The listing builds one solid part. Answer for the finished solid, in the listing's coordinates (mm). A direction names the side the tool comes from. Give positions to 0.01 mm unless a question says otherwise; leave off trailing zeros. Loops run counter-clockwise (first coordinate to the right, second up) from the corner with the lowest first, then second, coordinate; pieces in that order, holes last.
Item 1: The mould has two halves that part along X. Classify faces 3 (the face through (22, 79, -70.679)), 4 (the face through (12, 76.072, -67)): pulls with the +X half, pulls with the -X half, needs draft (parallel to the pull), parting line crosses it, or undercut.
Item 2: Section A-A, the plane x = -18 is taken. Give the vertices of the cut face in (y, z), and give its area (3 significant figures).
Item 3: Each of these flat-tipped pins is pushed along its axis until it touches: pin 1 Ø3 at (x, y) = (32.47, 78.92) entering from +Z; pin 2 Ø1.7 at (x, y) = (62.5, 80) entering from +Z; pin 3 Ø4 at (x, y) = (13.5, 78) entering from +Z. Where does it stop, or does it pass through?
Item 4: A tool of negligible diameter and unlimited length cuts with its end or side. For faces 1 (the face through (12.12, 77.31, -69.3)), 2 (the face through (32, 76.072, -67)), from which of +Z, -Z, +X, -X, +Y, -Y can it reach the whole face along a straight path? Write none if from no direction.
Item 5: Consider line 1 along X through (y, z) = (79.5, -65.9); line 2 along X through (y, z) = (79, -67.25); line 3 along Y through (x, z) = (11, -68.55). Determine where each line is inside the solid, lowest interval first.
from build123d import *

# Parameters (mm, degrees)
SKETCH1_W           = 99.9
SKETCH1_H           = 24.9
SKETCH1_R           = 1.65
BOSS_EXTRUDE1_DEPTH = 5
CUT_EXTRUDE1_DEPTH  = 2.2


with BuildPart() as part:
    # Sketch1 → Boss-Extrude1 (new body)
    with BuildSketch(Plane.XY.offset(-70.679368873)):
        with Locations((22.473815584, 78.921604181)):
            Rectangle(SKETCH1_W, SKETCH1_H)
        with Locations((-17.526184416, 78.921604181)):
            Circle(SKETCH1_R, mode=Mode.SUBTRACT)
        with Locations((12.473815584, 78.921604181)):
            Circle(SKETCH1_R, mode=Mode.SUBTRACT)
        with Locations((32.473815584, 78.921604181)):
            Circle(SKETCH1_R, mode=Mode.SUBTRACT)
        with Locations((62.473815584, 78.921604181)):
            Circle(SKETCH1_R, mode=Mode.SUBTRACT)
    extrude(amount=BOSS_EXTRUDE1_DEPTH)

    # Sketch2 → Cut-Extrude1 (cut)
    with BuildSketch(Plane.XY.offset(-65.679368873)):
        Polygon((-15.880736149, 76.071604181), (-14.235287881, 78.921604181), (-15.880736149, 81.771604181), (-19.171632683, 81.771604181), (-20.81708095, 78.921604181), (-19.171632683, 76.071604181), align=None)
        Polygon((14.119263851, 76.071604181), (15.764712119, 78.921604181), (14.119263851, 81.771604181), (10.828367317, 81.771604181), (9.18291905, 78.921604181), (10.828367317, 76.071604181), align=None)
        Polygon((34.119263851, 76.071604181), (35.764712119, 78.921604181), (34.119263851, 81.771604181), (30.828367317, 81.771604181), (29.18291905, 78.921604181), (30.828367317, 76.071604181), align=None)
        Polygon((64.119263851, 76.071604181), (65.764712119, 78.921604181), (64.119263851, 81.771604181), (60.828367317, 81.771604181), (59.18291905, 78.921604181), (60.828367317, 76.071604181), align=None)
    extrude(amount=-CUT_EXTRUDE1_DEPTH, mode=Mode.SUBTRACT)


solid = part.part
Worked answers:
1. face 3: needs draft
1. face 4: undercut
2. outline: (66.47, -70.68) - (77.34, -70.68) - (77.34, -67.88) - (76.07, -67.88) - (76.07, -65.68) - (66.47, -65.68) - close; (80.5, -70.68) - (91.37, -70.68) - (91.37, -65.68) - (81.77, -65.68) - (81.77, -67.88) - (80.5, -67.88) - close
2. area: 103 mm2
3. pin 1: passes through
3. pin 2: stops at z = -67.88
3. pin 3: stops at z = -65.68
4. face 1: +Z, -Z
4. face 2: +Z
5. line 1: x = -27.48 to -20.48, -14.57 to 9.52, 15.43 to 29.52, 35.43 to 59.52, 65.43 to 72.42
5. line 2: x = -27.48 to -20.77, -14.28 to 9.23, 15.72 to 29.23, 35.72 to 59.23, 65.72 to 72.42
5. line 3: y = 66.47 to 78.18, 79.66 to 91.37
